The listing builds one solid part. Answer for the finished solid, in the listing's coordinates (mm). Coordinates: 2 decimals unless noted, no trailing zeros. Order: outer loops, then holes, each group sorted by start corner. A loop starts at its lowest first (then second) coordinate and runs counter-clockwise, first axis right, second up. Notation, with made-up numbers: (77, 24.5) -> (95, 24.5) arc R13 ccw to (95, 32.5) -> close; hole circle Ø1 at (70, 50.5). An arc over 180 degrees is marked (long way). Return JSON: item names as keys, results as strings.
```python
from build123d import *

# Parameters (mm, degrees)
F0_R     = 1.5875
F1_DEPTH = 11.1125
F2_R     = 1.2065
F3_DEPTH = 0.508
F4_R     = 1.5875
F4_R_2   = 1.2065
F5_DEPTH = 1.27
F6_R     = 1.2065
F7_DEPTH = 0.508
F8_R     = 1.5875
F8_R_2   = 1.2065
F9_DEPTH = 1.27


with BuildPart() as f1:
    # F0 (on Front) → F1 (new body, symmetric)
    with BuildSketch(Plane.XZ):
        Circle(F0_R)
    extrude(amount=F1_DEPTH, both=True)

    # F2 (on face) → F3 (join)
    with BuildSketch(Plane.XZ.offset(11.1125)):
        Circle(F2_R)
    extrude(amount=F3_DEPTH)

    # F4 (on face) → F5 (join)
    with BuildSketch(Plane.XZ.offset(11.6205)):
        Circle(F4_R)
        Circle(F4_R_2, mode=Mode.SUBTRACT)
        Circle(F4_R_2)
    extrude(amount=F5_DEPTH)

    # F6 (on face) → F7 (join)
    with BuildSketch(Plane(origin=(0, 11.1125, 0), x_dir=(-1, 0, 0), z_dir=(0, 1, 0))):
        Circle(F6_R)
    extrude(amount=F7_DEPTH)

    # F8 (on face) → F9 (join)
    with BuildSketch(Plane(origin=(0, 11.6205, 0), x_dir=(-1, 0, 0), z_dir=(0, 1, 0))):
        Circle(F8_R)
        Circle(F8_R_2, mode=Mode.SUBTRACT)
        Circle(F8_R_2)
    extrude(amount=F9_DEPTH)


solid = f1.part
```
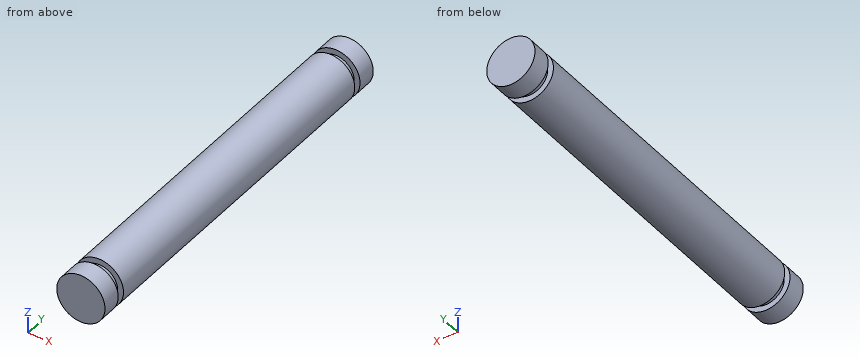
Item 1: The part is cut by section B-B on y = 7. Determine the outline of the cut face in (x, z) (1 decimal), plus the area to 3 significant figures.
Answer list:
{"outline": "circle Ø3.2 at (0, 0)", "area": "7.92 mm2"}
Item 2: Find the intervals of material crossed by probe 1 along Y at (x, z) = (0.25, -1.35); probe 2 along Z at (x, y) = (0.1, 7.5); probe 3 along X at (y, z) = (7.25, 0.85), in increasing order.
Answer list:
{"probe 1": "-12.89 to -11.62, -11.11 to 11.11, 11.62 to 12.89", "probe 2": "-1.58 to 1.58", "probe 3": "-1.34 to 1.34"}
Item 3: The part is cut by section A-A on x = 0.5. Determine the outline of the cut face in (y, z).
Answer list:
{"outline": "(-12.89, -1.51) -> (-11.62, -1.51) -> (-11.62, -1.1) -> (-11.11, -1.1) -> (-11.11, -1.51) -> (11.11, -1.51) -> (11.11, -1.1) -> (11.62, -1.1) -> (11.62, -1.51) -> (12.89, -1.51) -> (12.89, 1.51) -> (11.62, 1.51) -> (11.62, 1.1) -> (11.11, 1.1) -> (11.11, 1.51) -> (-11.11, 1.51) -> (-11.11, 1.1) -> (-11.62, 1.1) -> (-11.62, 1.51) -> (-12.89, 1.51) -> close"}
